```python
from build123d import *

# Parameters (mm, degrees)
RESSALTO_EXTRUS_O1_DEPTH  = 100
RESSALTO_EXTRUS_O2_DEPTH  = 100
ESBO_O3_W                 = 45
ESBO_O3_H                 = 1.5
RESSALTO_EXTRUS_O3_DEPTH  = 25
CORTE_EXTRUS_O1_DEPTH     = 104.630352696
ESBO_O5_W                 = 12
ESBO_O5_H                 = 1.5
CORTE_EXTRUS_O2_DEPTH     = 108.079409785
CORTE_EXTRUS_O3_DEPTH     = 108.439517869
RESSALTO_EXTRUS_O10_DEPTH = 26.5


with BuildPart() as part:
    # Esboço1 → Ressalto-extrusão1 (new body)
    with BuildSketch(Plane.XY):
        Polygon((-22.5, 12.5), (-22.5, -12.5), (22.5, -12.5), (22.5, 12.5), (24, 12.5), (24, -14), (-24, -14), (-24, 12.5), align=None)
    extrude(amount=RESSALTO_EXTRUS_O1_DEPTH)

    # Esboço2 → Ressalto-extrusão2 (add)
    with BuildSketch(Plane(origin=(0, 0, 0), x_dir=(-1, 0, 0), z_dir=(0, 0, -1))):
        Polygon((-24, 12.5), (-29, 12.5), (-29, 11.5), (-24, 6.5), align=None)
        Polygon((-24, 3.5), (-29, 3.5), (-29, 2.5), (-24, -2.5), align=None)
        Polygon((29, 3.5), (29, 2.5), (24, -2.5), (24, 3.5), align=None)
        Polygon((29, 12.5), (29, 11.5), (24, 6.5), (24, 12.5), align=None)
    extrude(amount=-RESSALTO_EXTRUS_O2_DEPTH)

    # Esboço3 → Ressalto-extrusão3 (add)
    with BuildSketch(Plane(origin=(0, -12.5, 0), x_dir=(1, 0, 0), z_dir=(0, 1, 0))):
        with Locations((0, -0.75)):
            Rectangle(ESBO_O3_W, ESBO_O3_H)
    extrude(amount=RESSALTO_EXTRUS_O3_DEPTH)

    # Esboço4 → Corte-extrusão1 (cut, through all)
    with BuildSketch(Plane.XY.offset(1.5)):
        Polygon((-10, -12.5), (10, -12.5), (10, -7.5), (5, -2.5), (-5, -2.5), (-10, -7.5), align=None)
    extrude(amount=-CORTE_EXTRUS_O1_DEPTH, mode=Mode.SUBTRACT)

    # Esboço5 → Corte-extrusão2 (cut, through all)
    with BuildSketch(Plane(origin=(0, -12.5, 0), x_dir=(1, 0, 0), z_dir=(0, 1, 0))):
        with Locations((0, -2.25)):
            Rectangle(ESBO_O5_W, ESBO_O5_H)
    extrude(amount=-CORTE_EXTRUS_O2_DEPTH, mode=Mode.SUBTRACT)

    # Esboço9 → Corte-extrusão3 (cut, through all)
    with BuildSketch(Plane.XZ.offset(14)):
        Polygon((-12.515135483, 96), (-29, 90), (-29, 100), (-12.515135483, 100), align=None)
        Polygon((29, 100), (29, 90), (12.515135483, 96), (12.515135483, 100), align=None)
    extrude(amount=-CORTE_EXTRUS_O3_DEPTH, mode=Mode.SUBTRACT)

    # Esboço6 → Ressalto-extrusão10 (add, through all)
    with BuildSketch(Plane.XZ.offset(14)):
        with BuildLine():
            Line((-6, 110), (6, 110))
            Line((6, 110), (6, 108.718795841))
            ThreePointArc((6, 108.718795841), (6.720673479, 106.132801926), (8.674945811, 104.292270904))
            ThreePointArc((8.674945811, 104.292270904), (9.598817012, 103.827932437), (10.538733862, 103.396997961))
            Line((10.538733862, 103.396997961), (12.600450366, 108.0363228))
            Line((12.600450366, 108.0363228), (13.247345381, 107.802907073))
            Line((13.247345381, 107.802907073), (13.247345381, 102.372045387))
            ThreePointArc((13.247345381, 102.372045387), (16.773859685, 101.477410085), (20.384927381, 101.033714749))
            ThreePointArc((20.384927381, 101.033714749), (21.87541452, 101.575227938), (22.50318548, 103.031487553))
            Line((22.50318548, 103.031487553), (22.501243671, 106.084324825))
            Line((22.501243671, 106.084324825), (28.501243671, 106.084324825))
            ThreePointArc((28.501243671, 106.084324825), (26.712485124, 101.810515585), (22.412761864, 100.08497728))
            ThreePointArc((22.412761864, 100.08497728), (13.860011295, 101.244470296), (6, 104.810166412))
            Line((6, 104.810166412), (6, 102.41442124))
            Line((6, 102.41442124), (11.616924727, 96.797496513))
            Line((11.616924727, 96.797496513), (11.616924727, 93.797496513))
            Line((11.616924727, 93.797496513), (-11.616924727, 93.797496513))
            Line((-11.616924727, 93.797496513), (-11.616924727, 96.797496513))
            Line((-11.616924727, 96.797496513), (-6, 102.41442124))
            Line((-6, 102.41442124), (-6, 104.810166412))
            ThreePointArc((-6, 104.810166412), (-13.860011295, 101.244470296), (-22.412761864, 100.08497728))
            ThreePointArc((-22.412761864, 100.08497728), (-26.712485124, 101.810515585), (-28.501243671, 106.084324825))
            Line((-28.501243671, 106.084324825), (-22.501243671, 106.084324825))
            Line((-22.501243671, 106.084324825), (-22.50318548, 103.031487553))
            ThreePointArc((-22.50318548, 103.031487553), (-21.87541452, 101.575227938), (-20.384927381, 101.033714749))
            ThreePointArc((-20.384927381, 101.033714749), (-16.773859685, 101.477410085), (-13.247345381, 102.372045387))
            Line((-13.247345381, 102.372045387), (-13.247345381, 107.802907073))
            Line((-13.247345381, 107.802907073), (-12.600450366, 108.0363228))
            Line((-12.600450366, 108.0363228), (-10.538733862, 103.396997961))
            ThreePointArc((-10.538733862, 103.396997961), (-9.598817012, 103.827932437), (-8.674945811, 104.292270904))
            ThreePointArc((-8.674945811, 104.292270904), (-6.720673479, 106.132801926), (-6, 108.718795841))
            Line((-6, 108.718795841), (-6, 110))
        make_face()
    extrude(amount=-RESSALTO_EXTRUS_O10_DEPTH)


solid = part.part
```
Geometry check sheet. Reference: the model listing, model coordinates, mm. A direction names the side the tool comes from. Give positions to 0.01 mm unless a question says otherwise; leave off trailing zeros. Order: outer loops, then holes, each group sorted by start corner. A loop starts at its lowest first (then second) coordinate and runs counter-clockwise, first axis right, second up.
1. Thickness scan on L1, parallel to X at y = -3.5, z = 76; L2, parallel to X at y = 11.75, z = 43; L3, parallel to Z at x = 2.5, y = 2.75. Record the ranges inside material, lowest first.
2. Section check C-C, the plane z = 30. Enter the section's corners in (x, y), and give its area (3 significant figures).
3. Section check B-B, the plane x = -17. Enter the section's corners in (y, z).
4. Section check A-A, the plane x = -2.5. Enter the section's corners in (y, z).
5. Release check for a two-part mould opening along X. For faces 4 (the face through (16.724, -0.935, 101.487)), 5 (the face through (0, 0, 93.797)), 6 (the face through (-11.584, -0.935, 105.749)), 7 (the face through (26.5, 9, 45.3)) record: pulls with the +X half, pulls with the -X half, needs draft (parallel to the pull), parting line crosses it, or undercut.
6. Gauge pin test, flat ends, axial feed: pin 1 Ø12.5 at (y, z) = (-10.5, 36) entering from -X; pin 2 Ø1.5 at (y, z) = (0, 94) entering from +X; pin 3 Ø0.8 at (y, z) = (-9, 1) entering from +X; pin 4 Ø7.5 at (y, z) = (5, 38.5) entering from -X. Record the tip position at first contact, or that the pin passes through.
7. Access from +Z, -Z, +X, -X, +Y, -Y to the whole of each face (thin tool, end or side, straight path). Record for faces 1 (the face through (26, 3.5, 45)), 2 (the face through (-11.617, 0, 95)), 3 (the face through (-16.82, -0.94, 101.47)).
Values follow:
1. L1: x = -24 to -22.5, 22.5 to 24
1. L2: x = -29 to -22.5, 22.5 to 29
1. L3: z = 0 to 1.5, 93.8 to 110
2. outline: (-29, 2.5) - (-24, -2.5) - (-24, -14) - (24, -14) - (24, -2.5) - (29, 2.5) - (29, 3.5) - (24, 3.5) - (24, 6.5) - (29, 11.5) - (29, 12.5) - (22.5, 12.5) - (22.5, -12.5) - (-22.5, -12.5) - (-22.5, 12.5) - (-29, 12.5) - (-29, 11.5) - (-24, 6.5) - (-24, 3.5) - (-29, 3.5) - close
2. area: 217 mm2
3. outline: (-14, 0) - (12.5, 0) - (12.5, 1.5) - (-12.5, 1.5) - (-12.5, 94.37) - (-14, 94.37) - close; (-14, 100.52) - (12.5, 100.52) - (12.5, 101.44) - (-14, 101.44) - close
4. outline: (-14, 0) - (-12.5, 0) - (-12.5, 1.5) - (-14, 1.5) - close; (-14, 3) - (-12.5, 3) - (-12.5, 93.8) - (12.5, 93.8) - (12.5, 110) - (-14, 110) - close; (-2.5, 0) - (12.5, 0) - (12.5, 1.5) - (-2.5, 1.5) - close
5. face 4: undercut
5. face 5: needs draft
5. face 6: undercut
5. face 7: pulls with the +X half
6. pin 1: stops at x = -24
6. pin 2: stops at x = 11.62
6. pin 3: stops at x = 24
6. pin 4: stops at x = -29
7. face 1: -Z, +X
7. face 2: -X, +Y
7. face 3: +Z, +Y, -Y
